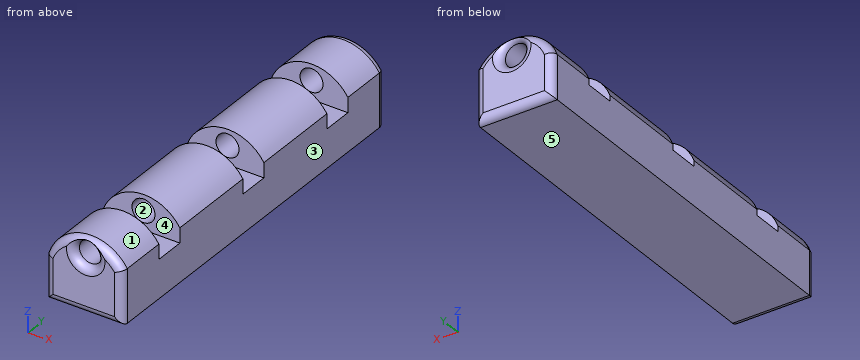
```python
from build123d import *

# Parameters (mm, degrees)
BOSS_EXTRUDE1_DEPTH     = 20
CUT_EXTRUDE1_DEPTH      = 5
SKETCH3_W               = 10
SKETCH3_H               = 50.00000000000001
CUT_EXTRUDE2_DEPTH      = 18.000000000000007
CUT_EXTRUDE3_DEPTH      = 45.955533585978046
CUT_EXTRUDE3_DEPTH_BACK = 45.955533585978046
SKETCH4_R               = 1.5
CUT_EXTRUDE4_DEPTH      = 55.772255750516614
CUT_EXTRUDE4_DEPTH_BACK = 55.772255750516614
FILLET1_R               = 1


with BuildPart() as part:
    # Sketch1 → Boss-Extrude1 (new body)
    with BuildSketch(Plane.XY):
        Polygon((0, 0), (10, 0), (10.000000000000007, -50), (6.12e-15, -50), align=None)
    extrude(amount=BOSS_EXTRUDE1_DEPTH)

    # Sketch2 → Cut-Extrude1 (cut)
    with BuildSketch(Plane.XY.offset(20)):
        Polygon((10.000000000000009, -7), (8.6e-16, -7), (7.6e-16, -11), (10.000000000000005, -11), align=None)
        Polygon((10.000000000000007, -23), (1.47e-15, -23), (3.8e-16, -27), (10.000000000000004, -27), align=None)
        Polygon((10.000000000000005, -39), (1.47e-15, -39), (0, -43), (10.000000000000007, -43), align=None)
    extrude(amount=-CUT_EXTRUDE1_DEPTH, mode=Mode.SUBTRACT)

    # Sketch3 → Cut-Extrude2 (cut)
    with BuildSketch(Plane(origin=(10, 1.39e-15, 0), x_dir=(0, 0, -1), z_dir=(1, 1.4e-16, 0))):
        with Locations((-5, -25.000000000000004)):
            Rectangle(SKETCH3_W, SKETCH3_H)
    extrude(amount=-CUT_EXTRUDE2_DEPTH, mode=Mode.SUBTRACT)

    # Sketch4 → Cut-Extrude3 (cut, two sides: drawn at the far end of the back side and taken through both)
    with BuildSketch(Plane.XZ.offset(39).offset(-CUT_EXTRUDE3_DEPTH_BACK)):
        with Locations(Location((5.260991578815225, 17.426547092913836, 0), (0, 0, 270))):
            Circle(SKETCH4_R)
    extrude(amount=CUT_EXTRUDE3_DEPTH + CUT_EXTRUDE3_DEPTH_BACK, mode=Mode.SUBTRACT)

    # Sketch5 → Cut-Extrude4 (cut, two sides: drawn at the far end of the back side and taken through both)
    with BuildSketch(Plane.XZ.offset(50).offset(-CUT_EXTRUDE4_DEPTH_BACK)):
        with BuildLine():
            Line((6.12e-15, 20), (0, 15.73755811618498))
            ThreePointArc((-8.9e-16, 15.73755811618498), (4.6252026328097955, 19.461842499702882), (10.000000000000007, 16.93709561624879))
            Line((10.000000000000007, 16.93709561624879), (10.000000000000007, 20))
            Line((10.000000000000007, 20), (6.12e-15, 20))
        make_face()
    extrude(amount=CUT_EXTRUDE4_DEPTH + CUT_EXTRUDE4_DEPTH_BACK, mode=Mode.SUBTRACT)

    # Fillet1
    # the kernel refuses this fillet: 1 mm, written as the material it takes off along each edge
    with BuildSketch(Plane(origin=(10, 0, 7.5), x_dir=(-1, 0, 0), z_dir=(0, 0, 1))) as fillet1_piece_1:
        with BuildLine():
            CenterArc((FILLET1_R, FILLET1_R), FILLET1_R, 180, 90)
            Line((0, FILLET1_R), (0, 0))
            Line((0, 0), (FILLET1_R, 0))
        make_face()
    extrude(amount=11.93709561624879, mode=Mode.SUBTRACT)
    with BuildSketch(Plane(origin=(0, 0, 7.5), x_dir=(1, 0, 0), z_dir=(0, 0, 1))) as fillet1_piece_2:
        with BuildLine():
            CenterArc((FILLET1_R, -FILLET1_R), FILLET1_R, 90, 90)
            Line((2.2e-16, -FILLET1_R), (0, 0))
            Line((0, 0), (FILLET1_R, 0))
        make_face()
    extrude(amount=10.737558116184978, mode=Mode.SUBTRACT)
    with BuildSketch(Plane(origin=(6.12e-15, -50, 7.5), x_dir=(-1.3e-16, 1, 0), z_dir=(0, 0, 1))) as fillet1_piece_3:
        with BuildLine():
            CenterArc((FILLET1_R, -FILLET1_R), FILLET1_R, 90, 89.99999999999997)
            Line((-1.3e-16, -FILLET1_R), (0, 0))
            Line((0, 0), (FILLET1_R, 0))
        make_face()
    extrude(amount=10.737558116184978, mode=Mode.SUBTRACT)
    with BuildSketch(Plane(origin=(10.000000000000007, -50, 7.5), x_dir=(0, 1, 0), z_dir=(0, 0, 1))) as fillet1_piece_4:
        with BuildLine():
            CenterArc((FILLET1_R, FILLET1_R), FILLET1_R, 180, 90)
            Line((0, FILLET1_R), (0, 0))
            Line((0, 0), (FILLET1_R, 0))
        make_face()
    extrude(amount=11.93709561624879, mode=Mode.SUBTRACT)
    with BuildSketch(Plane(origin=(5.292490697981418, -50, 13.898964597710425), x_dir=(-0.9937101746292788, 0, -0.11198253809522406), z_dir=(0.11198253809522406, 0, -0.9937101746292788))) as fillet1_piece_5:
        with BuildLine():
            CenterArc((5.602756813783422 - FILLET1_R, FILLET1_R), FILLET1_R, 270, 90)
            Line((5.602756813783423, FILLET1_R), (5.602756813783422, 0))
            Line((5.602756813783422, 0), (5.602756813783422 - FILLET1_R, 0))
        make_face()
    revolve(axis=Axis((5.292490697981418, -50, 13.898964597710425), (0, 1, 0)), revolution_arc=179.17890353520545, mode=Mode.SUBTRACT)
    with BuildSketch(Plane(origin=(5.292490697981418, 0, 13.898964597710425), x_dir=(-0.9937101746292788, 0, -0.11198253809522406), z_dir=(0.11198253809522406, 0, -0.9937101746292788))) as fillet1_piece_6:
        with BuildLine():
            CenterArc((5.602756813783421 - FILLET1_R, -FILLET1_R), FILLET1_R, 0, 90)
            Line((5.602756813783421, -FILLET1_R), (5.602756813783421, 0))
            Line((5.602756813783421, 0), (5.602756813783421 - FILLET1_R, 0))
        make_face()
    revolve(axis=Axis((5.292490697981418, 0, 13.898964597710425), (0, 1, 0)), revolution_arc=179.17890353520545, mode=Mode.SUBTRACT)
    with BuildSketch(Plane(origin=(12.500000000000007, -50, 10), x_dir=(-1.4e-16, 1, 0), z_dir=(-1, -1.4e-16, 0))) as fillet1_piece_7:
        with BuildLine():
            CenterArc((FILLET1_R, -FILLET1_R), FILLET1_R, 90, 90)
            Line((0, -FILLET1_R), (0, 0))
            Line((0, 0), (FILLET1_R, 0))
        make_face()
    extrude(amount=15.000000000000002, mode=Mode.SUBTRACT)
    with BuildSketch(Plane(origin=(12.5, 0, 10), x_dir=(0, 0, 1), z_dir=(-1, -1.4e-16, 0))) as fillet1_piece_8:
        with BuildLine():
            CenterArc((FILLET1_R, -FILLET1_R), FILLET1_R, 90, 90)
            Line((0, -FILLET1_R), (0, 0))
            Line((0, 0), (FILLET1_R, 0))
        make_face()
    extrude(amount=15, mode=Mode.SUBTRACT)
    with BuildSketch(Plane(origin=(5.260991578815225, 0, 17.426547092913836), x_dir=(0, 0, -1), z_dir=(-1, 0, 0))) as fillet1_piece_9:
        with BuildLine():
            CenterArc((1.5 + FILLET1_R, FILLET1_R), FILLET1_R, 180, 90)
            Line((1.5, FILLET1_R), (1.5, 0))
            Line((1.5, 0), (1.5 + FILLET1_R, 0))
        make_face()
    revolve(axis=Axis((5.260991578815225, 0, 17.426547092913836), (0, -1, 0)), mode=Mode.SUBTRACT)
    with BuildSketch(Plane(origin=(5.260991578815225, -50, 17.426547092913836), x_dir=(0, 0, -1), z_dir=(1, 0, 0))) as fillet1_piece_10:
        with BuildLine():
            CenterArc((1.5 + FILLET1_R, FILLET1_R), FILLET1_R, 180, 90)
            Line((1.5, FILLET1_R), (1.5, 0))
            Line((1.5, 0), (1.5 + FILLET1_R, 0))
        make_face()
    revolve(axis=Axis((5.260991578815225, -50, 17.426547092913836), (0, 1, 0)), mode=Mode.SUBTRACT)


solid = part.part
```
Read the model definition and answer for the solid it produces. Units are mm, in the model's axes. Face numbers are marked on the shaded views. A direction names the side the tool comes from. Give positions to 0.01 mm unless a question says otherwise; leave off trailing zeros. Order: outer loops, then holes, each group sorted by start corner. A loop starts at its lowest first (then second) coordinate and runs counter-clockwise, first axis right, second up.
(1) Find section D-D (y = -26). Give the vertices of the cut face in (x, z), plus the area to 3 significant figures.
(2) Find section B-B (y = -19.5). Give the vertices of the cut face in (x, z), plus the area to 3 significant figures.
(3) For the marked faces 4 and 5, determine the directions among +Z, -Z, +X, -X, +Y, -Y from which every point of the face is accessible in a straight line to the end or side of a thin tool.
(4) For a pull along Z with two mould halves and no side action, classify the marked faces 1, 2 and 3 as released by +Z, released by -Z, zero draft, split by the parting line, or undercut.
(5) Find section A-A (z = 18.5). Give the number of separate pieces and of enclosed holes in the cut face, plus the area to 3 significant figures.
(6) Straight lines are drawn through the part: L1, parallel to Y at x = 1, z = 15.75; L2, parallel to Z at x = 2.5, y = -25.5; L3, parallel to Z at x = 5, y = -20. For each, find the intervals that lie inside material, in ascending order.
(7) Given pin 1 (1.2 mm diameter, centred on x = 3.5, y = -9.5, fed in from +Z); pin 2 (4 mm diameter, centred on x = 5.26, z = 17.43, fed in from -Y); pin 3 (4 mm diameter, centred on x = 5.26, z = 17.43, fed in from +Y), each flat-ended and moving along its own axis, determine where each tip first touches the part or whether it passes through.
Result sheet:
1. outline: (0, 10) - (10, 10) - (10, 15) - (0, 15) - close
1. area: 50.0 mm2
2. outline: (0, 10) - (10, 10) - (10, 16.94) arc R5.6 ccw to (0, 15.74) - close; hole circle Ø3 at (5.26, 17.43)
2. area: 79.0 mm2
3. face 4: +Z, +X, -X
3. face 5: -Z, +X, -X, +Y, -Y
4. face 1: released by +Z
4. face 2: undercut
4. face 3: zero draft
5. separate pieces: 8
5. enclosed holes: 0
5. area: 161 mm2
6. L1: y = -50 to -43, -39 to -27, -23 to -11, -7 to 0
6. L2: z = 10 to 15
6. L3: z = 10 to 15.95, 18.9 to 19.49
7. pin 1: stops at z = 15
7. pin 2: stops at y = -49.87
7. pin 3: stops at y = -0.13
